Geometry: final body of the model. Coordinates: model frame, mm. A direction names the side the tool comes from. Coordinates: 2 decimals unless noted, no trailing zeros. Order: outer loops, then holes, each group sorted by start corner. A loop starts at its lowest first (then second) coordinate and runs counter-clockwise, first axis right, second up. Notation, with made-up numbers: (10.25, -10.75) -> (24.25, -10.75) arc R25 cw to (24.25, 22.25) -> close; hole circle Ø9 at (57, 21). An arc over 180 degrees is marked (long way). Use one line per item in the form item = value.
```python
from build123d import *

# Parameters (mm, degrees)
SKETCH_1_R             = 37
SKETCH_1_W             = 100
SKETCH_1_H             = 3
EXTRUDE_1_DEPTH        = 44
SKETCH_2_R             = 34
CUT_EXTRUDE_1_DEPTH    = 40
SKETCH_4_R             = 1.6
CUT_EXTRUDE_2_DEPTH    = 10
PATTERN_LINEAR_1_COUNT = 2
PATTERN_LINEAR_1_PITCH = 90


with BuildPart() as part:
    # ｽｹｯﾁ1 → ﾎﾞｽ - 押し出し1 (new body)
    with BuildSketch(Plane.XY):
        with Locations((-5.795339113, 4.185414542)):
            Circle(SKETCH_1_R)
        with Locations((-5.795339113, 41.771570891)):
            Rectangle(SKETCH_1_W, SKETCH_1_H)
    extrude(amount=EXTRUDE_1_DEPTH)

    # ｽｹｯﾁ2 → ｶｯﾄ - 押し出し1 (cut)
    with BuildSketch(Plane(origin=(0, 0, 0), x_dir=(-1, 0, 0), z_dir=(0, 0, -1))):
        with Locations((5.795339113, 4.185414542)):
            Circle(SKETCH_2_R)
    extrude(amount=-CUT_EXTRUDE_1_DEPTH, mode=Mode.SUBTRACT)

    # ｽｹｯﾁ4 → ｶｯﾄ - 押し出し2 (cut)
    with BuildSketch(Plane(origin=(0, 43.271570891, 0), x_dir=(1, 0, 0), z_dir=(0, 1, 0))):
        with Locations((-50.795339113, -5)):
            Circle(SKETCH_4_R)
        with Locations((-50.795339113, -15)):
            Circle(SKETCH_4_R)
        with Locations((-50.795339113, -25)):
            Circle(SKETCH_4_R)
        with Locations((-50.795339113, -35)):
            Circle(SKETCH_4_R)
    cut_extrude_2 = extrude(amount=-CUT_EXTRUDE_2_DEPTH, mode=Mode.SUBTRACT)

    # 直線ﾊﾟﾀｰﾝ1: ｶｯﾄ - 押し出し2 ×2
    with Locations(*[(i * PATTERN_LINEAR_1_PITCH, 0, 0) for i in range(1, PATTERN_LINEAR_1_COUNT)]):
        add(cut_extrude_2, mode=Mode.SUBTRACT)


solid = part.part
```
1) Section A-A, the plane z = 25. Output: boundary loops of the cut face in (x, y), and give its area (3 significant figures).
Results found:
outline = (-55.8, 40.27) -> (-52.4, 40.27) -> (-52.4, 43.27) -> (-55.8, 43.27) -> close; (-49.2, 40.27) -> (-13.97, 40.27) arc R37 ccw (long way) to (2.38, 40.27) -> (37.6, 40.27) -> (37.6, 43.27) -> (-49.2, 43.27) -> close; (40.8, 40.27) -> (44.2, 40.27) -> (44.2, 43.27) -> (40.8, 43.27) -> close; hole circle Ø68 at (-5.8, 4.19)
area = 940 mm2
2) Section D-D, the plane z = 20. Output: boundary loops of the cut face in (x, y).
Results found:
outline = (-55.8, 40.27) -> (-13.97, 40.27) arc R37 ccw (long way) to (2.38, 40.27) -> (44.2, 40.27) -> (44.2, 43.27) -> (-55.8, 43.27) -> close; hole circle Ø68 at (-5.8, 4.19)
3) Pull-direction query (Y, two-part tool) for faces 1 (the flat face through (-6, 43.272, 22)), 2 (the cylindrical face through (-7.307, -32.784, 21.692)), 3 (the cylindrical face through (37.93, 41.79, 35.97)); classes: released by +Y, released by -Y, zero draft, split by the parting line, or undercut.
Results found:
face_1 = released by +Y
face_2 = undercut
face_3 = zero draft
4) Contact query for flat-ended pins moving along their axis: P1, Ø8, axis at y = 18.5, z = 25.5, coming from the -X side; P2, Ø1, axis at y = -12, z = 27.5, coming from the -X side; P3, Ø4, axis at x = 39.2, z = 5, coming from the -Y side; P4, Ø1.9, axis at x = -50.8, z = 25, coming from the -Y side. Output: stop coordinate, or through.
Results found:
P1 = -41.33
P2 = -39.31
P3 = 40.27
P4 = through
5) Section B-B, the plane x = 17.5. Output: boundary loops of the cut face in (y, z).
Results found:
outline = (-24.56, 0) -> (-20.58, 0) -> (-20.58, 40) -> (28.95, 40) -> (28.95, 0) -> (32.93, 0) -> (32.93, 44) -> (-24.56, 44) -> close; (40.27, 0) -> (43.27, 0) -> (43.27, 44) -> (40.27, 44) -> close
6) Access query for faces 4 (the flat face through (-6, 39, 0)), 5 (the flat face through (-35, 40.272, 22)), 6 (the flat face through (23, 40.272, 22)), 7 (the flat face through (-6, 6, 44)), 8 (the flat face through (-5, 5, 40)). Directions: +Z, -Z, +X, -X, +Y, -Y. A direction counts if a zero-diameter tool reaches every point of the face in a straight line with its end or side. Return the directions, or none.
Results found:
face_4 = -Z, +X, -X, +Y, -Y
face_5 = +Z, -Z, -X
face_6 = +Z, -Z, +X
face_7 = +Z, +X, -X, +Y, -Y
face_8 = -Z
7) Section C-C, the plane y = -3. Output: boundary loops of the cut face in (x, z), and give its area (3 significant figures).
Results found:
outline = (-42.09, 0) -> (-39.03, 0) -> (-39.03, 40) -> (27.44, 40) -> (27.44, 0) -> (30.5, 0) -> (30.5, 44) -> (-42.09, 44) -> close
area = 535 mm2
8) Material intervals for probe 1 along X at (y, z) = (42, 15); probe 2 along Y at (x, z) = (5.5, 20.5); probe 3 along X at (y, z) = (4, 34.5), sorted ascending. Write a range as from..to.
Results found:
probe_1 = -55.8..-52.4, -49.2..37.6, 40.8..44.2
probe_2 = -31.05..-27.88, 36.25..39.42, 40.27..43.27
probe_3 = -42.79..-39.79, 28.2..31.2
